from build123d import *

# Parameters (mm, degrees)
BOSS_EXTRUDE1_DEPTH  = 19
FILLET1_R            = 10
BOSS_EXTRUDE2_DEPTH  = 19
SKETCH2_R            = 14.5
CUT_EXTRUDE1_DEPTH   = 20
M5_CLEARANCE_HOLE2_D = 5.5
M5_CLEARANCE_HOLE1_D = 5.5
M5_CLEARANCE_HOLE3_D = 5.5
M8_CLEARANCE_HOLE1_D = 9
CUT_EXTRUDE2_DEPTH   = 4
CUT_EXTRUDE3_DEPTH   = 4
SKETCH16_R           = 19.05
CUT_EXTRUDE4_DEPTH   = 2
CUT_EXTRUDE5_DEPTH   = 20


# Read off the part's stored shape, not the designer's step: Boss-Extrude2
with BuildPart() as part:
    # Sketch1 → Boss-Extrude1 (new body)
    with BuildSketch(Plane.XY):
        with BuildLine():
            Line((-170.200000001, 540.824594888), (-129.309401077, 470))
            Line((-129.309401077, 470), (-93, 470))
            ThreePointArc((-93, 470), (-90.878679656, 470.878679656), (-90, 473))
            Line((-90, 473), (-90, 564.25527297))
            Line((-90, 564.25527297), (-116.225329238, 607))
            Line((-116.225329238, 607), (-170.200000001, 607))
            Line((-170.200000001, 607), (-170.200000001, 540.824594888))
        make_face()
    extrude(amount=BOSS_EXTRUDE1_DEPTH)

    # Fillet1
    fillet1_edges = [part.edges().sort_by_distance(p)[0] for p in [
        (-90, 564.25527297, 9.5),
        (-129.309401077, 470, 9.5),
        (-170.200000001, 540.824594888, 9.5),
    ]]
    fillet(fillet1_edges, radius=FILLET1_R)

    # Boss-Extrude2 outline → Boss-Extrude2 (add)
    with BuildSketch(Plane.XY):
        with BuildLine():
            Line((-93, 470), (-90, 470))
            ThreePointArc((-90, 470), (-82.928932188, 472.928932188), (-80, 480))
            Line((-80, 480), (-80, 561.432106106))
            ThreePointArc((-80, 561.432106106), (-80.75234172, 566.866041212), (-82.952765074, 571.89115871))
            Line((-82.952765074, 571.89115871), (-106.530973281, 610.321336823))
            ThreePointArc((-106.530973281, 610.321336823), (-111.626593598, 615.216765438), (-118.464037729, 617))
            Line((-118.464037729, 617), (-166.200000001, 617))
            ThreePointArc((-166.200000001, 617), (-176.099494937, 612.899494936), (-180.200000001, 603))
            Line((-180.200000001, 603), (-180.200000001, 543.504086813))
            ThreePointArc((-180.200000001, 543.504086813), (-179.518516526, 538.327705911), (-177.520508076, 533.504086813))
            Line((-177.520508076, 533.504086813), (-143.743157806, 475))
            ThreePointArc((-143.743157806, 475), (-140.082903769, 471.339745962), (-135.082903769, 470))
            Line((-135.082903769, 470), (-123.535898385, 470))
            ThreePointArc((-123.535898385, 470), (-128.535898385, 471.339745962), (-132.196152423, 475))
            Line((-132.196152423, 475), (-168.860254039, 538.504086813))
            ThreePointArc((-168.860254039, 538.504086813), (-169.859258264, 540.915896362), (-170.200000001, 543.504086813))
            Line((-170.200000001, 543.504086813), (-170.200000001, 607))
            Line((-170.200000001, 607), (-116.225329238, 607))
            Line((-116.225329238, 607), (-91.476382537, 566.661632408))
            ThreePointArc((-91.476382537, 566.661632408), (-90.37617086, 564.149073659), (-90, 561.432106106))
            Line((-90, 561.432106106), (-90, 473))
            ThreePointArc((-90, 473), (-90.878679656, 470.878679656), (-93, 470))
        make_face()
    extrude(amount=BOSS_EXTRUDE2_DEPTH)

    # Sketch2 → Cut-Extrude1 (cut)
    with BuildSketch(Plane.XY.offset(19)):
        with Locations((-140, 577)):
            Circle(SKETCH2_R)
    extrude(amount=-CUT_EXTRUDE1_DEPTH, mode=Mode.SUBTRACT)

    # M5 Clearance Hole2 (through all)
    with Locations(Plane(origin=(0, 0, 0), x_dir=(-1, 0, 0), z_dir=(0, 0, -1))):
        with Locations((117.000000001, 595), (117.000000001, 577), (163.000000001, 577), (163.000000001, 595)):
            Hole(M5_CLEARANCE_HOLE2_D / 2)

    # M5 Clearance Hole1 (through all)
    with Locations(Plane.XY.offset(19)):
        with Locations((-95, 545), (-125, 545), (-125, 475), (-95, 475), (-110, 490), (-110, 530)):
            Hole(M5_CLEARANCE_HOLE1_D / 2)

    # M5 Clearance Hole3 (through all)
    with Locations(Plane.XY.offset(19)):
        with Locations((-140.000000001, 543.666986335), (-173.333013666, 577), (-106.666986336, 577), (-140.000000001, 610.333013665)):
            Hole(M5_CLEARANCE_HOLE3_D / 2)

    # M8 Clearance Hole1 (through all)
    with Locations(Plane(origin=(-110, 490, 0), x_dir=(-1, 0, 0), z_dir=(0, 0, -1))):
        with Locations((0, 0), (0, 40)):
            Hole(M8_CLEARANCE_HOLE1_D / 2)

    # Sketch14 → Cut-Extrude2 (cut)
    with BuildSketch(Plane(origin=(0, 0, 19), x_dir=(-1, 0, 0), z_dir=(0, 0, -1))):
        Polygon((117.000000001, 581.572614132), (113.04, 579.286307066), (113.04, 574.713692934), (117.000000001, 572.427385868), (120.960000001, 574.713692934), (120.960000001, 579.286307066), align=None)
        Polygon((163.000000001, 581.572614133), (159.04, 579.286307066), (159.04, 574.713692934), (163.000000001, 572.427385867), (166.960000001, 574.713692934), (166.960000001, 579.286307066), align=None)
        Polygon((163.000000001, 599.572614132), (159.040000001, 597.286307066), (159.040000001, 592.713692934), (163.000000001, 590.427385868), (166.960000001, 592.713692934), (166.960000001, 597.286307066), align=None)
        Polygon((120.960000001, 597.286307066), (117.000000001, 599.572614132), (113.040000001, 597.286307066), (113.040000001, 592.713692934), (117.000000001, 590.427385868), (120.960000001, 592.713692934), align=None)
    extrude(amount=CUT_EXTRUDE2_DEPTH, mode=Mode.SUBTRACT)

    # Sketch15 → Cut-Extrude3 (cut)
    with BuildSketch(Plane.XY):
        Polygon((-143.233326461, 546.900312795), (-144.416806085, 542.483506711), (-141.183479624, 539.25018025), (-136.76667354, 540.433659874), (-135.583193916, 544.850465958), (-138.816520377, 548.083792419), align=None)
        Polygon((-143.233326462, 613.566340126), (-144.416806085, 609.149534041), (-141.183479624, 605.91620758), (-136.76667354, 607.099687204), (-135.583193916, 611.516493288), (-138.816520377, 614.749819749), align=None)
        Polygon((-109.900312796, 580.23332646), (-111.083792419, 575.816520376), (-107.850465959, 572.583193916), (-103.433659875, 573.766673539), (-102.250180252, 578.183479623), (-105.483506712, 581.416806083), align=None)
        Polygon((-172.149534042, 581.416806083), (-176.566340126, 580.23332646), (-177.749819749, 575.816520376), (-174.516493289, 572.583193916), (-170.099687205, 573.766673539), (-168.916207582, 578.183479623), align=None)
    extrude(amount=CUT_EXTRUDE3_DEPTH, mode=Mode.SUBTRACT)

    # Sketch16 → Cut-Extrude4 (cut)
    with BuildSketch(Plane.XY.offset(19)):
        with Locations((-140, 577)):
            Circle(SKETCH16_R)
    extrude(amount=-CUT_EXTRUDE4_DEPTH, mode=Mode.SUBTRACT)

    # Sketch17 → Cut-Extrude5 (cut)
    with BuildSketch(Plane.XY.offset(19)):
        Polygon((-148.25, 540.1), (-148.25, 519.9), (-143.533578644, 519.9), (-139.608578644, 523.825), (-137.641421356, 523.825), (-133.716421356, 519.9), (-130, 519.9), (-130, 540.1), (-133.716421356, 540.1), (-137.641421356, 536.175), (-139.608578644, 536.175), (-143.533578644, 540.1), align=None)
    extrude(amount=-CUT_EXTRUDE5_DEPTH, mode=Mode.SUBTRACT)


solid = part.part
Model file for the job. Use its own axes, mm. A direction names the side the tool comes from. Coordinates: 2 decimals unless noted, no trailing zeros. Order: outer loops, then holes, each group sorted by start corner. A loop starts at its lowest first (then second) coordinate and runs counter-clockwise, first axis right, second up. Notation, with made-up numbers: (63.25, -19.75) -> (90.25, -19.75) arc R26 cw to (90.25, 13.25) -> close; hole circle Ø11 at (28.5, 54.5). An arc over 180 degrees is marked (long way). Return JSON: item names as keys, results as strings. Group by question number.
Item 1: Flat gauge pins, fed straight in: P1, Ø4.5, axis at y = 595, z = 16.5, coming from the +X side; P2, Ø1, axis at x = -117, z = 9.5, coming from the +Y side; P3, Ø2, axis at y = 577, z = 17, coming from the +X side. Where does each tip first touch, or does it go through?
Item 2: Pull direction X, two halves, no side cores. Call faces 1 (the cylindrical face through (-150.687, 586.8, 8.619)), 2 (the flat face through (-131, 545, 0)), 3 (the flat face through (-180.2, 574, 9)): pulls with the +X half, pulls with the -X half, needs draft (parallel to the pull), parting line crosses it, or undercut.
Item 3: Wall check: line 1 along Y through (x, z) = (-95, 12); line 2 along X through (y, z) = (577, 10.25); line 3 along Y through (x, z) = (-163, 6.5). Give the ranges that are in metal, low to high. Write a range as [from, to].
Item 4: Saw through at B-B on y = 530. Write the cut outline in (x, z).
Item 5: Tool access for faces 4 (the flat face through (-142.823, 607.556, 1.972)), 5 (the flat face through (-132, 540.1, 10)), 6 (the flat face through (-133, 590, 17)): list every direction of +Z, -Z, +X, -X, +Y, -Y with a clear straight run to the whole face (end or side of a thin tool).
Item 6: Saw through at D-D on x = -131.5. Write the cut outline in (y, z).
Item 7: Saw through at A-A on x = -151. Write the cut outline in (y, z).
Item 8: Saw through at C-C on z = 1.75. State how many separate pieces and enclosed holes the cut face has, then the cut area to 3 significant figures.
Values found:
{
 "1": {"P1": "stops at x = -95.75", "P2": "stops at y = 616.97", "P3": "stops at x = -85.47"},
 "2": {"face 1": "undercut", "face 2": "needs draft", "face 3": "pulls with the -X half"},
 "3": {"line 1": "y = [470, 472.25], [477.75, 542.25], [547.75, 591.53]", "line 2": "x = [-180.2, -176.08], [-170.58, -165.75], [-160.25, -154.5], [-125.5, -119.75], [-114.25, -109.42], [-103.92, -86.09]", "line 3": "y = [508.35, 574.25], [579.75, 592.25], [597.75, 617]"},
 "4": {"outline": "(-175.5, 0) -> (-148.25, 0) -> (-148.25, 19) -> (-175.5, 19) -> close; (-130, 0) -> (-114.5, 0) -> (-114.5, 19) -> (-130, 19) -> close; (-105.5, 0) -> (-80, 0) -> (-80, 19) -> (-105.5, 19) -> close"},
 "5": {"face 4": "-Z", "face 5": "+Z, -Z", "face 6": "+Z"},
 "6": {"outline": "(470, 0) -> (519.9, 0) -> (519.9, 19) -> (470, 19) -> close; (540.1, 0) -> (565.25, 0) -> (565.25, 17) -> (559.95, 17) -> (559.95, 19) -> (540.1, 19) -> close; (588.75, 0) -> (617, 0) -> (617, 19) -> (594.05, 19) -> (594.05, 17) -> (588.75, 17) -> close"},
 "7": {"outline": "(487.57, 0) -> (567.55, 0) -> (567.55, 17) -> (561.45, 17) -> (561.45, 19) -> (487.57, 19) -> close; (586.45, 0) -> (617, 0) -> (617, 19) -> (592.55, 19) -> (592.55, 17) -> (586.45, 17) -> close"},
 "8": {"separate pieces": "1", "enclosed holes": "16", "area": "11,000 mm2"}
}
